Build history of the part. All positions in model axes, mm. A direction names the side the tool comes from. Coordinates: 2 decimals unless noted, no trailing zeros. Order: outer loops, then holes, each group sorted by start corner. A loop starts at its lowest first (then second) coordinate and runs counter-clockwise, first axis right, second up. Notation, with made-up numbers: (-6.75, 6.25) - (32.25, 6.25) arc R8 ccw to (32.25, 20.25) - close; hole circle Ø1 at (89.25, 55). An arc over 180 degrees is marked (long way). Answer as CSV lines item,"result". Start each with the question number.
from build123d import *

# Parameters (mm, degrees)
SKETCH_1_R      = 1.5
SKETCH_1_R_2    = 7.2
EXTRUDE_1_DEPTH = 3


with BuildPart() as part:
    # 草图1 → 凸台-拉伸1 (new body)
    with BuildSketch(Plane(origin=(0, 0, 0), x_dir=(1, 0, 0), z_dir=(0, 1, 0))):
        with BuildLine():
            Line((-58.582677165, 11.57480315), (-6.889301028, 11.57480315))
            ThreePointArc((-6.889301028, 11.57480315), (14.417322835, 1.57480315), (-6.889301028, -8.42519685))
            Line((-6.889301028, -8.42519685), (-58.582677165, -8.42519685))
            Line((-58.582677165, -8.42519685), (-58.582677165, 11.57480315))
        make_face()
        with Locations((-33.582677165, 7.57480315)):
            Circle(SKETCH_1_R, mode=Mode.SUBTRACT)
        with Locations((-48.582677165, 7.57480315)):
            Circle(SKETCH_1_R, mode=Mode.SUBTRACT)
        with Locations((-33.582677165, -4.42519685)):
            Circle(SKETCH_1_R, mode=Mode.SUBTRACT)
        with Locations((-48.582677165, -4.42519685)):
            Circle(SKETCH_1_R, mode=Mode.SUBTRACT)
        with Locations((1.417322835, 1.57480315)):
            Circle(SKETCH_1_R_2, mode=Mode.SUBTRACT)
        with Locations((10.917322835, 1.57480315)):
            Circle(SKETCH_1_R, mode=Mode.SUBTRACT)
        with Locations((-3.332677165, -6.652438186)):
            Circle(SKETCH_1_R, mode=Mode.SUBTRACT)
        with Locations((-3.332677165, 9.802044486)):
            Circle(SKETCH_1_R, mode=Mode.SUBTRACT)
    extrude(amount=EXTRUDE_1_DEPTH)


solid = part.part
(1) Probe L1, parallel to X at y = 0.55, z = 3.75; L2, parallel to X at y = 0.7, z = -1.75; L3, parallel to X at y = 2.35, z = -6.5. List the from-to ranges inside material, lowest first. Write a range as [from, to].
(2) Drop flat-ended pins along their axis: pin 1 Ø2.5 at (x, z) = (-3.33, 6.65) entering from +Y; pin 2 Ø1 at (x, y) = (-16, 2) entering from -Z. Give the stop position or say it passes through.
(3) Band-saw the part on C-C on y = 2.2. State how many separate pieces and enclosed holes the cut face has, plus the area to 3 significant figures.
(4) Which spindle directions (+Z, -Z, +X, -X, +Y, -Y) get a long thin tool onto all of the face, cutting with end or side? Do faces 1 (the flat face through (-32, 1, 8.425)), 2 (the cylindrical face through (-47.78, 1.48, -8.84)), 3 (the flat face through (-33, 1, -11.575)). Say none if no direction does.
(5) Band-saw the part on B-B on z = 7.5. List the corners of the cut face in (x, y).
(6) Pull direction Z, two halves, no side cores. Call faces 4 (the cylindrical face through (-33.78, 1.48, -9.06)), 5 (the cylindrical face through (12.303, 1.479, -1)), 6 (the flat face through (-58.583, 1, -1)), 7 (the cylindrical face through (14.41, 1.48, -1.99)): +Z half, -Z half, draft (parallel to the pull), parting line (faces both ways), or undercut.
(7) Band-saw the part on A-A on x = 4. List the corners of the cut face in (y, z), plus the area to 3 significant figures.
(8) Band-saw the part on D-D on x = -52.5. List the corners of the cut face in (y, z).
Filled in:
1,L1,"x = [-58.58, -49.92], [-47.24, -34.92], [-32.24, -3.43], [6.26, 13.28]"
1,L2,"x = [-58.58, -5.78], [8.62, 9.43], [12.41, 14.42]"
1,L3,"x = [-58.58, -49.63], [-47.54, -34.63], [-32.54, -3.83], [6.67, 13.45]"
2,pin 1,"passes through"
2,pin 2,"stops at z = -11.57"
3,separate pieces,"1"
3,enclosed holes,"8"
3,area,"1,290 mm^2"
4,face 1,"+Z, -X, +Y, -Y"
4,face 2,"+Y, -Y"
4,face 3,"-Z, -X, +Y, -Y"
5,outline,"(-58.58, 0) - (-4.57, 0) - (-4.57, 3) - (-58.58, 3) - close; (-2.1, 0) - (10.73, 0) - (10.73, 3) - (-2.1, 3) - close"
6,face 4,"undercut"
6,face 5,"undercut"
6,face 6,"draft"
6,face 7,"parting line"
7,outline,"(0, -14.32) - (3, -14.32) - (3, -8.3) - (0, -8.3) - close; (0, 5.15) - (3, 5.15) - (3, 11.17) - (0, 11.17) - close"
7,area,"36.1 mm^2"
8,outline,"(0, -11.57) - (3, -11.57) - (3, 8.43) - (0, 8.43) - close"
